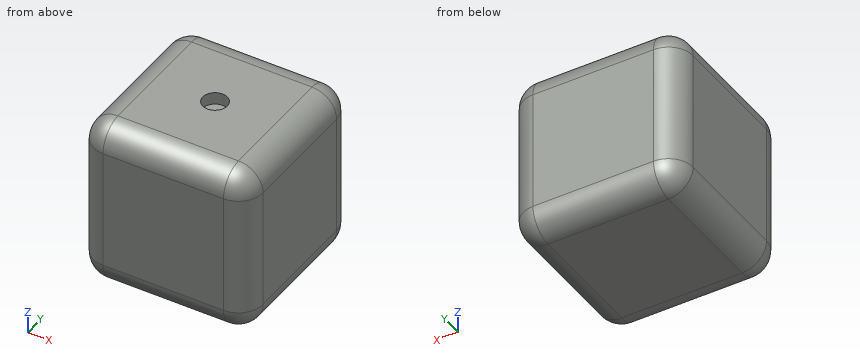
from build123d import *

# Parameters (mm, degrees)
F0_W     = 17.526
F0_H     = 17.526
F1_DEPTH = 17.526
F2_R     = 2.54
F3_R     = 1.27
F4_DEPTH = 1.27


with BuildPart() as f1:
    # F0 (on Top) → F1 (new body)
    with BuildSketch(Plane.XY):
        with Locations((8.763, 8.763)):
            Rectangle(F0_W, F0_H)
    extrude(amount=F1_DEPTH)

    # F2
    f2_edges = [f1.edges().sort_by_distance(p)[0] for p in [
        (0, 8.763, 17.526),
        (8.763, 0, 17.526),
        (17.526, 8.763, 17.526),
        (8.763, 17.526, 17.526),
        (0, 0, 8.763),
        (17.526, 0, 8.763),
        (8.763, 0, 0),
        (17.526, 17.526, 8.763),
        (17.526, 8.763, 0),
        (0, 17.526, 8.763),
        (0, 8.763, 0),
        (8.763, 17.526, 0),
    ]]
    fillet(f2_edges, radius=F2_R)

    # F3 (on face) → F4 (cut)
    with BuildSketch(Plane.XY.offset(17.526)):
        with Locations((8.763, 8.763)):
            Circle(F3_R)
    extrude(amount=-F4_DEPTH, mode=Mode.SUBTRACT)


solid = f1.part
Verification items for the finished model (mm, model axes). Give positions to 0.01 mm unless a question says otherwise; leave off trailing zeros. Order: outer loops, then holes, each group sorted by start corner. A loop starts at its lowest first (then second) coordinate and runs counter-clockwise, first axis right, second up. Notation, with made-up numbers: M -13,7.5 L 21,7.5 A14 cw 21,29.5 Z; hole C 12,16.5 d3. An arc over 180 degrees is marked long. Answer as a JSON object with one key per item and string values. Group by question number.
1) Cross-section at C-C (x = 8). Enter the section's corners in (y, z), then the cut area to 3 significant figures.
2) Scan lines: line 1 along Y through (x, z) = (8.75, 17.25); line 2 along Z through (x, y) = (16.25, 12.75); line 3 along Z through (x, y) = (16.5, 8.75). Record each from-to range of solid material in increasing order. Write a range as [from, to].
3) Cross-section at A-A (y = 11.75). Enter the section's corners in (x, z), then the cut area to 3 significant figures.
Result sheet:
{
 "1": {"outline": "M 0,2.54 A2.54 ccw 2.54,0 L 14.99,0 A2.54 ccw 17.53,2.54 L 17.53,14.99 A2.54 ccw 14.99,17.53 L 9.78,17.53 L 9.78,16.26 L 7.75,16.26 L 7.75,17.53 L 2.54,17.53 A2.54 ccw 0,14.99 Z", "area": "299 mm2"},
 "2": {"line 1": "y = [1.39, 7.49], [10.03, 16.14]", "line 2": "z = [0.34, 17.19]", "line 3": "z = [0.5, 17.03]"},
 "3": {"outline": "M 0,2.54 A2.54 ccw 2.54,0 L 14.99,0 A2.54 ccw 17.53,2.54 L 17.53,14.99 A2.54 ccw 14.99,17.53 L 2.54,17.53 A2.54 ccw 0,14.99 Z", "area": "302 mm2"}
}
